```python
from build123d import *

# Parameters (mm, degrees)
F0_R     = 10.16
F1_DEPTH = 3.8608
F2_R     = 6.35
F3_DEPTH = 15.24
F4_R     = 1.3081
F5_DEPTH = 3.8608
F6_R     = 3.3909
F7_DEPTH = 19.1008


with BuildPart() as f1:
    # F0 (on Top) → F1 (new body)
    with BuildSketch(Plane.XY):
        Circle(F0_R)
    extrude(amount=F1_DEPTH)

    # F2 (on face) → F3 (join)
    with BuildSketch(Plane.XY.offset(3.8608)):
        Circle(F2_R)
    extrude(amount=F3_DEPTH)

    # F4 (on face) → F5 (cut, through all)
    with BuildSketch(Plane.XY.offset(3.8608)):
        with BuildLine():
            ThreePointArc((0, 6.9469), (0.924966, 7.330034), (1.3081, 8.255))
            ThreePointArc((1.3081, 8.255), (0.924966, 9.179966), (0, 9.5631))
            Line((0, 9.5631), (0, 6.9469))
        make_face()
        with BuildLine():
            Line((0, 6.9469), (0, 9.5631))
            ThreePointArc((0, 9.5631), (-1.3081, 8.255), (0, 6.9469))
        make_face()
        with Locations((-7.14904, -4.1275)):
            Circle(F4_R)
        with Locations((7.14904, -4.1275)):
            Circle(F4_R)
    extrude(amount=-F5_DEPTH, mode=Mode.SUBTRACT)

    # F6 (on face) → F7 (cut, through all)
    with BuildSketch(Plane.XY.offset(19.1008)):
        Circle(F6_R)
    extrude(amount=-F7_DEPTH, mode=Mode.SUBTRACT)


solid = f1.part
```
Check sheet for the modelled part. Datum: model origin and axes. Units: mm. A direction names the side the tool comes from. Coordinates: 2 decimals unless noted, no trailing zeros. Order: outer loops, then holes, each group sorted by start corner. A loop starts at its lowest first (then second) coordinate and runs counter-clockwise, first axis right, second up. Notation, with made-up numbers: (59.25, 6) -> (92.25, 6) arc R26 cw to (92.25, 35) -> close; hole circle Ø4 at (14.25, 17). An arc over 180 degrees is marked (long way). Write item = value, one per line. Start each with the question number.
1) Cross-section at A-A (y = 0). Enter the section's corners in (x, z), then the cut area to 3 significant figures.
2) Cross-section at D-D (z = 13). Enter the section's corners in (x, y).
3) Cross-section at B-B (z = 3). Enter the section's corners in (x, y) (1 decimal), then the cut area to 3 significant figures.
4) Mould release check, pull along Y, two halves, no side actions. Record for faces 3 (the flat face through (3, -3, 19.101)), 4 (the cylindrical face through (3.234, 1.019, 9.684)), 5 (the cylindrical face through (6.185, -3.243, 1.957)), 6 (the cylindrical face through (-1.38, -6.2, 11.37)): +Y half, -Y half, draft (parallel to the pull), parting line (faces both ways), or undercut.
5) Material ranges on L1, parallel to Y at x = 0, z = 8.75; L2, parallel to Z at x = 7, y = 6.75; L3, parallel to Y at x = 2.75, z = 16.5, recorded low to high.
6) Cross-section at C-C (x = -4). Enter the section's corners in (y, z), then the cut area to 3 significant figures.
7) Access from +Z, -Z, +X, -X, +Y, -Y to the whole of each face (thin tool, end or side, straight path). Record for faces 1 (the flat face through (0, -7, 3.861)), 2 (the cylindrical face through (-6.45, -3.02, 1.96)).
8) Go/stop test with flat-tipped pins: P1, Ø6, axis at y = -5, z = 4, coming from the -X side; P2, Ø4, axis at x = 7.15, y = -4.13, coming from the +Z side; P3, Ø5, axis at y = 6.5, z = 17, coming from the -X side; P4, Ø6, axis at x = 5.5, z = 13.5, coming from the -Y side. Record where each tip stops, or that it passes through.
Ans:
q1.outline = (-10.16, 0) -> (-3.39, 0) -> (-3.39, 19.1) -> (-6.35, 19.1) -> (-6.35, 3.86) -> (-10.16, 3.86) -> close; (3.39, 0) -> (10.16, 0) -> (10.16, 3.86) -> (6.35, 3.86) -> (6.35, 19.1) -> (3.39, 19.1) -> close
q1.area = 142 mm²
q2.outline = circle Ø12.7 at (0, 0); hole circle Ø6.78 at (0, 0)
q3.outline = circle Ø20.3 at (0, 0); hole circle Ø2.6 at (-7.1, -4.1); hole circle Ø6.8 at (0, 0); hole (0, 6.9) arc R1.3 ccw to (1.3, 8.3) arc R1.3 ccw to (0, 9.6) arc R1.3 ccw to start; hole circle Ø2.6 at (7.1, -4.1)
q3.area = 272 mm²
q4.face_3 = draft
q4.face_4 = undercut
q4.face_5 = undercut
q4.face_6 = parting line
q5.L1 = -6.35 to -3.39, 3.39 to 6.35
q5.L2 = 0 to 3.86
q5.L3 = -5.72 to -1.98, 1.98 to 5.72
q6.outline = (-9.34, 0) -> (9.34, 0) -> (9.34, 3.86) -> (4.93, 3.86) -> (4.93, 19.1) -> (-4.93, 19.1) -> (-4.93, 3.86) -> (-9.34, 3.86) -> close
q6.area = 222 mm²
q7.face_1 = +Z
q7.face_2 = +Z, -Z
q8.P1 = -9.96
q8.P2 = 19.1
q8.P3 = -4.93
q8.P4 = -5.84
